Design review of the part built by this model. Coordinates are the model's own, in mm. Face numbers are marked on the shaded views. A direction names the side the tool comes from. Coordinates: 2 decimals unless noted, no trailing zeros. Loops run counter-clockwise (first coordinate to the right, second up) from the corner with the lowest first, then second, coordinate; pieces in that order, holes last.
Q1. For P1, Ø8, axis at x = 45, y = -162.5, coming from the -Z side; P2, Ø5, axis at x = 13.5, z = 5.5, coming from the -Y side; P3, Ø3, axis at y = -13, z = -4, coming from the -X side; P4, Ø1.5, axis at x = 75, z = -3.5, coming from the -Y side, all flat-tipped, find the tip position at first contact; note any pin that passes through.
Q2. Machinability: for the marked faces 1, 2 and 3, which of the approach directions +Z, -Z, +X, -X, +Y, -Y give a long, thin tool a straight path to every point of the face, cutting with its end or side? Answer none if there is none.
Q3. Add section A-A on y = -162.5. Give the boundary of the cut face in (x, z), and give its area (3 significant figures).
Q4. Add section C-C on y = -65.5. Give the boundary of the cut face in (x, z).
Q5. Add section B-B on x = 19.5. Give the boundary of the cut face in (y, z), and give its area (3 significant figures).
Q6. Draft analysis for pull direction Y (two halves, no side actions). For the marked faces 4, 5 and 6, state which applies: released by +Y, released by -Y, zero draft, split by the parting line, or undercut.
Q7. Wall thickness on probe 1 along Y at (x, z) = (45.75, 0); probe 2 along Y at (x, z) = (41, 0.75); probe 3 along Z at (x, y) = (40, 14.75): over which ranges is each line inside the solid? List them lowest first.
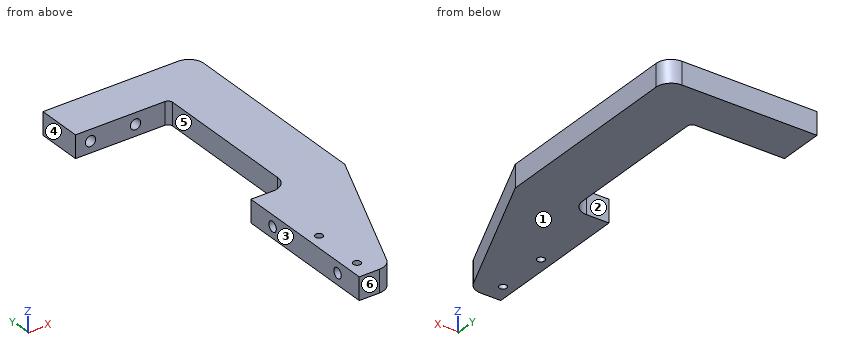
```python
from build123d import *

# Parameters (mm, degrees)
EXTRUDE_1_DEPTH        = 7.5
HOLE_WIZARD_M8_1_D     = 6.8
HOLE_WIZARD_M8_1_DEPTH = 19.75
HOLE_WIZARD_M8_1_TIP   = 2.042926105
HOLE_WIZARD_M8_2_D     = 6.8
HOLE_WIZARD_M8_2_DEPTH = 19.75
HOLE_WIZARD_M8_2_TIP   = 2.042926105
FILLET_1_R             = 10
FILLET_2_R             = 3
HOLE_WIZARD_M6_1_D     = 5


with BuildPart() as part:
    # 草图1 → 凸台-拉伸1 (new body, symmetric)
    with BuildSketch(Plane.XY):
        with BuildLine():
            Line((0, 0), (0, 30))
            Line((0, 30), (90, 30))
            ThreePointArc((90, 30), (97.071067812, 27.071067812), (100, 20))
            Line((100, 20), (100, -110))
            Line((100, -110), (57.5, -210))
            Line((57.5, -210), (37.5, -210))
            Line((37.5, -210), (37.5, -110))
            Line((37.5, -110), (62.5, -110))
            Line((62.5, -110), (62.5, 0))
            Line((62.5, 0), (0, 0))
        make_face()
    extrude(amount=EXTRUDE_1_DEPTH, both=True)

    # M8 螺纹孔1
    with Locations(Plane(origin=(0, 0, 0), x_dir=(-1, 0, 0), z_dir=(0, -1, 0))):
        with Locations((-40, 0), (-10, 0)):
            Hole(HOLE_WIZARD_M8_1_D / 2, depth=HOLE_WIZARD_M8_1_DEPTH)
            with Locations((0, 0, -(HOLE_WIZARD_M8_1_DEPTH + HOLE_WIZARD_M8_1_TIP / 2))):  # 118° drill point
                Cone(0, HOLE_WIZARD_M8_1_D / 2, HOLE_WIZARD_M8_1_TIP, mode=Mode.SUBTRACT)

    # M8 螺纹孔2
    with Locations(Plane.ZY.offset(-37.5)):
        with Locations((0, -130), (0, -190)):
            Hole(HOLE_WIZARD_M8_2_D / 2, depth=HOLE_WIZARD_M8_2_DEPTH)
            with Locations((0, 0, -(HOLE_WIZARD_M8_2_DEPTH + HOLE_WIZARD_M8_2_TIP / 2))):  # 118° drill point
                Cone(0, HOLE_WIZARD_M8_2_D / 2, HOLE_WIZARD_M8_2_TIP, mode=Mode.SUBTRACT)

    # 圆角1
    fillet_1_edges = [part.edges().sort_by_distance(p)[0] for p in [
        (57.5, -210, 0),
        (62.5, -110, 0),
    ]]
    fillet(fillet_1_edges, radius=FILLET_1_R)

    # 圆角2
    fillet_2_edges = [part.edges().sort_by_distance(p)[0] for p in [
        (62.5, 0, 0),
    ]]
    fillet(fillet_2_edges, radius=FILLET_2_R)

    # M6 螺纹孔1 (through all)
    with Locations(Plane(origin=(45, -162.5, 7.5), x_dir=(1, 0, 0), z_dir=(0, 0, 1))):
        with Locations((0, 0), (0, -35)):
            Hole(HOLE_WIZARD_M6_1_D / 2)


solid = part.part
```
Entries:
1. P1: stops at z = -7.5
1. P2: stops at y = 0
1. P3: stops at x = 62.5
1. P4: stops at y = -170.59
2. face 1: -Z, +X, -X, +Y, -Y
2. face 2: +Z, -Z, -X
2. face 3: +Z, -Z, -X, -Y
3. outline: (37.5, -7.5) - (42.5, -7.5) - (42.5, 7.5) - (37.5, 7.5) - close; (47.5, -7.5) - (77.69, -7.5) - (77.69, 7.5) - (47.5, 7.5) - close
3. area: 528 mm2
4. outline: (62.5, -7.5) - (100, -7.5) - (100, 7.5) - (62.5, 7.5) - close
5. outline: (0, -7.5) - (30, -7.5) - (30, 7.5) - (0, 7.5) - close
5. area: 450 mm2
6. face 4: zero draft
6. face 5: undercut
6. face 6: released by -Y
7. probe 1: y = -210 to -199.88, -195.12 to -193.4, -186.6 to -164.88, -160.12 to -133.4, -126.6 to -110, 0 to 30
7. probe 2: y = -210 to -193.32, -186.68 to -133.32, -126.68 to -110, 21.04 to 30
7. probe 3: z = -7.5 to -3.4, 3.4 to 7.5
